Answer from the drawing. Dimensions are ordinates in mm from the lowest x, y and z of the part. Round coordinates to 2 decimals unless told otherwise and drop trailing zeros. Loops run counter-clockwise (first coordinate to the right, second up) from the corner with the lowest first, then second, coordinate; pieces in that order, holes last.
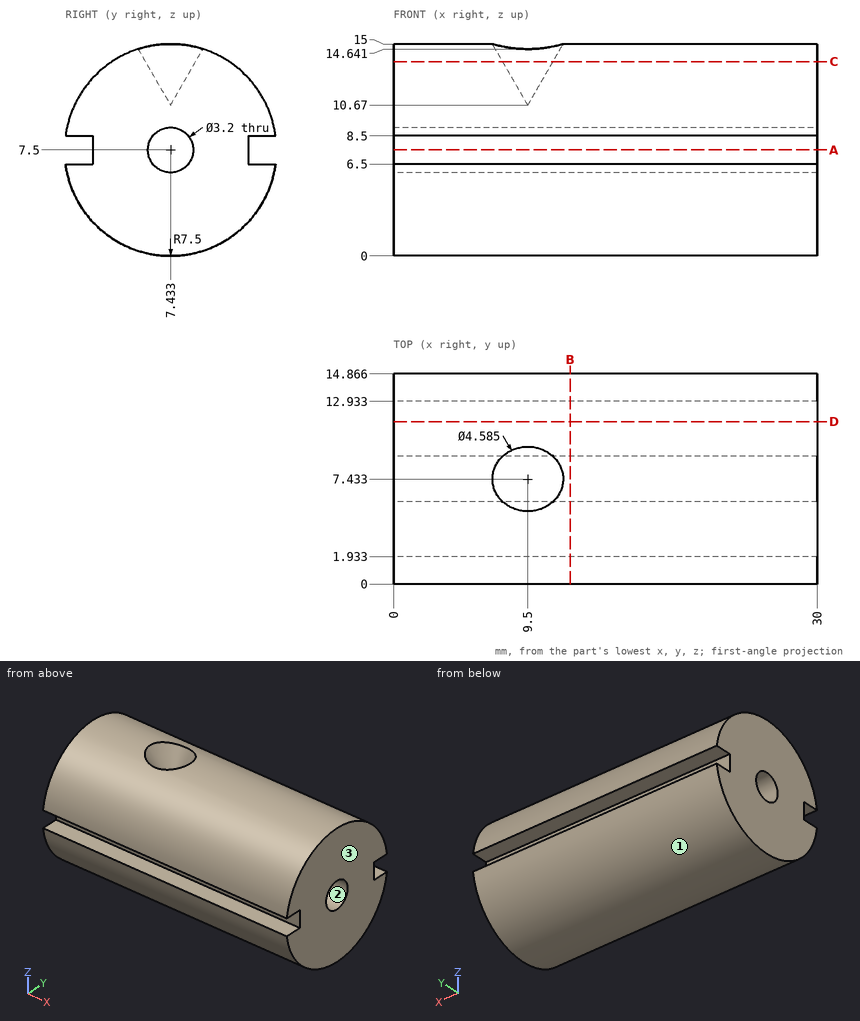
Item 1: Section B-B, the plane x = 12.5 is taken. Give the vertices of the cut face in (y, z).
Item 2: Straight lines are drawn through the part: line 1 (Y direction, x = 24, z = 7.5); line 2 (Y direction, x = 17, z = 7); line 3 (Z direction, x = 27.5, y = 6) (1 decimal). For each, find the intervals that lie inside material, in ascending order.
Item 3: Section C-C, the plane z = 13.75 is taken. Give the vertices of the cut face in (x, y) (1 decimal).
Item 4: Section A-A, the plane z = 7.5 is taken. Give the vertices of the cut face in (x, y), plus the area to 3 significant figures.
Item 5: Each of these flat-tipped pins is pushed along its axis until it touches: P1, Ø1, axis at x = 14, y = 1.5, coming from the -Z side; P2, Ø1.5, axis at x = 4, z = 7.5, coming from the -Y side; P3, Ø2, axis at x = 3, z = 2, coming from the -Y side. Where does it stop, or does it pass through?
Item 6: Section D-D, the plane y = 11.5 is taken. Give the vertices of the cut face in (x, z).
Item 7: Determine the mould class of the marked faces 1, 2 and 3 for opening direction Y: pulls with the +Y half, pulls with the -Y half, needs draft (parallel to the pull), parting line crosses it, or undercut.
Answer below:
1. outline: (0, 6.5) arc R7.5 ccw to (14.87, 6.5) - (12.93, 6.5) - (12.93, 8.5) - (14.87, 8.5) arc R7.5 ccw to (0, 8.5) - (1.93, 8.5) - (1.93, 6.5) - close; hole circle Ø3.2 at (7.43, 7.5)
2. line 1: y = 1.93 to 5.83, 9.03 to 12.93
2. line 2: y = 1.93 to 5.91, 8.95 to 12.93
2. line 3: z = 0.1 to 6.8, 8.2 to 14.9
3. outline: (0, 3.3) - (30, 3.3) - (30, 11.6) - (0, 11.6) - close; hole circle Ø3.6 at (9.5, 7.4)
4. outline: (0, 1.93) - (30, 1.93) - (30, 5.83) - (0, 5.83) - close; (0, 9.03) - (30, 9.03) - (30, 12.93) - (0, 12.93) - close
4. area: 234 mm2
5. P1: stops at z = 2.33
5. P2: stops at y = 1.93
5. P3: stops at y = 1.43
6. outline: (0, 1.2) - (30, 1.2) - (30, 13.8) - (0, 13.8) - close
7. face 1: parting line crosses it
7. face 2: undercut
7. face 3: needs draft
